Drawing for the job (mm, zero at the part's lowest x, y, z). A direction names the side the tool comes from. Give positions to 0.01 mm unless a question says otherwise; leave off trailing zeros. Order: outer loops, then holes, each group sorted by start corner. A loop starts at its lowest first (then second) coordinate and runs counter-clockwise, first axis right, second up. Notation, with made-up numbers: (83, 23) -> (113, 23) arc R24 ccw to (113, 39) -> close; hole circle Ø3 at (24, 67). An arc over 180 degrees is marked (long way). One line per item, written item: value. Start each with the question number.
(1) Probe line 1 (Z direction, x = 37, y = 27.75); line 2 (Y direction, x = 37, z = 3.5); line 3 (Y direction, x = 18, z = 4). List the from-to ranges inside material, lowest first.
(2) Saw through at B-B on y = 24. Give the cut face in (x, z), plus the area to 3 significant figures.
(3) Two-plate mould, pull along X, no slides. Class the marked faces 3, 4 and 5: +X half, -X half, draft (parallel to the pull), parting line (faces both ways), or undercut.
(4) Pin check, flat tip, straight feed: pin 1 (4 mm diameter, centred on x = 38.5, y = 18, fed in from +Z). Stop position of the tip, or through.
(5) Which spindle directions (+Z, -Z, +X, -X, +Y, -Y) get a long thin tool onto all of the face, cutting with end or side? Do the marked faces 1 and 2. Say none if no direction does.
(6) Saw through at C-C on z = 9.5. Give the cut face in (x, y), plus the area to 3 significant figures.
(7) Saw through at A-A on x = 37. Give the cut face in (y, z).
(8) Saw through at D-D on y = 18. Give the cut face in (x, z), plus the area to 3 significant figures.
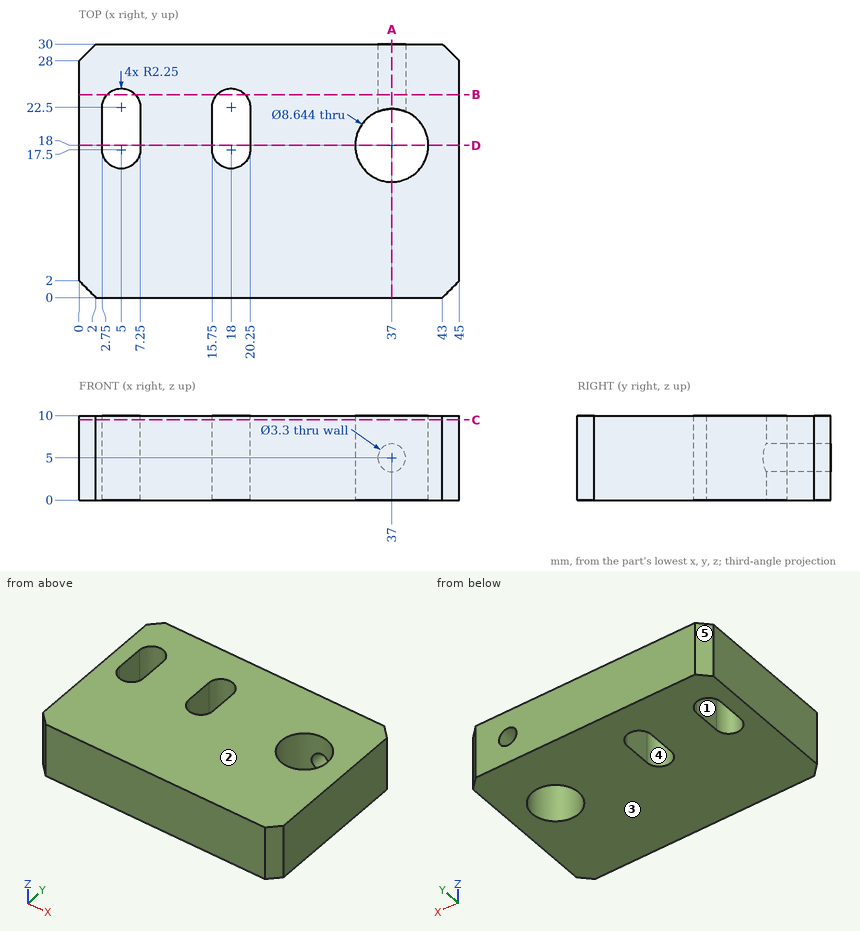
Results below:
1. line 1: z = 0 to 3.35, 6.65 to 10
1. line 2: y = 0 to 13.68
1. line 3: y = 0 to 15.25, 24.75 to 30
2. outline: (0, 0) -> (3.32, 0) -> (3.32, 10) -> (0, 10) -> close; (6.68, 0) -> (16.32, 0) -> (16.32, 10) -> (6.68, 10) -> close; (19.68, 0) -> (45, 0) -> (45, 10) -> (19.68, 10) -> close; hole circle Ø3.3 at (37, 5)
2. area: 374 mm²
3. face 3: draft
3. face 4: undercut
3. face 5: -X half
4. pin 1: passes through
5. face 1: +Z, -Z
5. face 2: +Z, +X, -X, +Y, -Y
6. outline: (0, 2) -> (2, 0) -> (43, 0) -> (45, 2) -> (45, 28) -> (43, 30) -> (2, 30) -> (0, 28) -> close; hole (2.75, 17.5) arc R2.25 ccw to (7.25, 17.5) -> (7.25, 22.5) arc R2.25 ccw to (2.75, 22.5) -> close; hole (15.75, 17.5) arc R2.25 ccw to (20.25, 17.5) -> (20.25, 22.5) arc R2.25 ccw to (15.75, 22.5) -> close; hole circle Ø8.64 at (37, 18)
6. area: 1,210 mm²
7. outline: (0, 0) -> (13.68, 0) -> (13.68, 10) -> (0, 10) -> close; (22.32, 0) -> (30, 0) -> (30, 3.35) -> (22.32, 3.35) -> close; (22.32, 6.65) -> (30, 6.65) -> (30, 10) -> (22.32, 10) -> close
8. outline: (0, 0) -> (2.75, 0) -> (2.75, 10) -> (0, 10) -> close; (7.25, 0) -> (15.75, 0) -> (15.75, 10) -> (7.25, 10) -> close; (20.25, 0) -> (32.68, 0) -> (32.68, 10) -> (20.25, 10) -> close; (41.32, 0) -> (45, 0) -> (45, 10) -> (41.32, 10) -> close
8. area: 274 mm²
